from build123d import *

# Parameters (mm, degrees)
BOSS_EXTRUDE1_DEPTH = 76.2
CUT_EXTRUDE1_START  = -3.175
SKETCH2_R           = 3.175
SKETCH2_R_2         = 2.921
CUT_EXTRUDE1_DEPTH  = 0.7874
CUT_EXTRUDE2_START  = -28.321
SKETCH3_R           = 3.175
SKETCH3_R_2         = 2.921
CUT_EXTRUDE2_DEPTH  = 0.7874
CUT_EXTRUDE3_START  = -22.8092
SKETCH3_6_R         = 3.175
SKETCH3_6_R_2       = 2.921
CUT_EXTRUDE3_DEPTH  = 0.7874
CUT_EXTRUDE4_START  = -6.1214
SKETCH3_7_R         = 3.175
SKETCH3_7_R_2       = 2.921
CUT_EXTRUDE4_DEPTH  = 0.7874


with BuildPart() as part:
    # Sketch1 → Boss-Extrude1 (new body)
    with BuildSketch(Plane(origin=(0, 0, 0), x_dir=(1, 0, 0), z_dir=(0, 1, 0))):
        with BuildLine():
            Line((-1, 3.01340754), (-1, 1.81340754))
            Line((-1, 1.81340754), (1, 1.81340754))
            Line((1, 1.81340754), (1, 3.01340754))
            ThreePointArc((1, 3.01340754), (0, -3.175), (-1, 3.01340754))
        make_face()
    extrude(amount=BOSS_EXTRUDE1_DEPTH)

    # Sketch2 → Cut-Extrude1 (cut)
    with BuildSketch(Plane(origin=(0, 76.2, 0), x_dir=(1, 0, 0), z_dir=(0, 1, 0)).offset(CUT_EXTRUDE1_START)):
        Circle(SKETCH2_R)
        Circle(SKETCH2_R_2, mode=Mode.SUBTRACT)
    extrude(amount=CUT_EXTRUDE1_DEPTH, mode=Mode.SUBTRACT)

    # Sketch3 → Cut-Extrude2 (cut)
    with BuildSketch(Plane(origin=(0, 0, 0), x_dir=(0, 0, -1), z_dir=(0, -1, 0)).offset(CUT_EXTRUDE2_START)):
        Circle(SKETCH3_R)
        Circle(SKETCH3_R_2, mode=Mode.SUBTRACT)
    extrude(amount=CUT_EXTRUDE2_DEPTH, mode=Mode.SUBTRACT)

    # Sketch3<6> → Cut-Extrude3 (cut)
    with BuildSketch(Plane(origin=(0, 0, 0), x_dir=(0, 0, -1), z_dir=(0, -1, 0)).offset(CUT_EXTRUDE3_START)):
        Circle(SKETCH3_6_R)
        Circle(SKETCH3_6_R_2, mode=Mode.SUBTRACT)
    extrude(amount=CUT_EXTRUDE3_DEPTH, mode=Mode.SUBTRACT)

    # Sketch3<7> → Cut-Extrude4 (cut)
    with BuildSketch(Plane(origin=(0, 0, 0), x_dir=(0, 0, -1), z_dir=(0, -1, 0)).offset(CUT_EXTRUDE4_START)):
        Circle(SKETCH3_7_R)
        Circle(SKETCH3_7_R_2, mode=Mode.SUBTRACT)
    extrude(amount=CUT_EXTRUDE4_DEPTH, mode=Mode.SUBTRACT)


solid = part.part
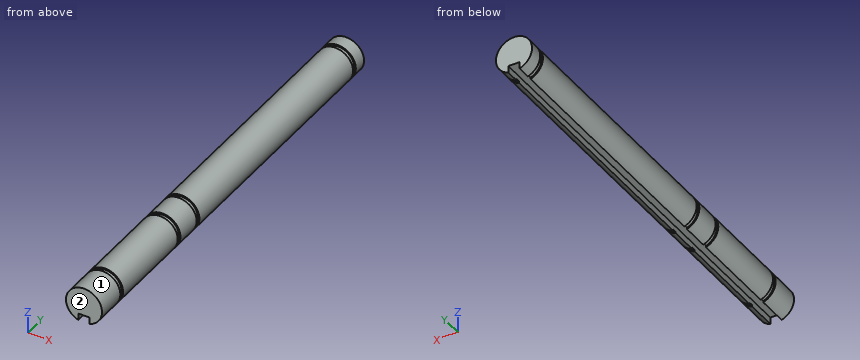
For this review, take the finished solid that the model builds, in its own axes (mm). Face numbers are marked on the shaded views. Coordinates: 2 decimals unless noted, no trailing zeros. Loops run counter-clockwise (first coordinate to the right, second up) from the corner with the lowest first, then second, coordinate; pieces in that order, holes last. Notation, with made-up numbers: (89, 19) - (100, 19) arc R30 ccw to (100, 55) - close; hole circle Ø7 at (31, 87.25). An arc over 180 degrees is marked (long way). Return JSON: item names as keys, results as strings.
Item 1: Insertion check: pin 1 (1.5 mm diameter, centred on x = 2, y = 16.5, fed in from -Z); pin 2 (1.6 mm diameter, centred on x = -0.5, y = 35, fed in from -Z); pin 3 (0.6 mm diameter, centred on y = 45, z = -2.5, fed in from +X). Each pin has a flat end and moves straight along its axis. Give the tip position at first contact, or say it passes through.
Determined:
{"pin 1": "stops at z = -2.92", "pin 2": "stops at z = -3.01", "pin 3": "stops at x = 2.29"}
Item 2: Take a section at A-A (x = 0). Give the boundary of the cut face in (y, z) (3 decimals), then the cut area to 3 significant figures.
Determined:
{"outline": "(0, -1.813) - (76.2, -1.813) - (76.2, 3.175) - (73.812, 3.175) - (73.812, 2.921) - (73.025, 2.921) - (73.025, 3.175) - (28.321, 3.175) - (28.321, 2.921) - (27.534, 2.921) - (27.534, 3.175) - (22.809, 3.175) - (22.809, 2.921) - (22.022, 2.921) - (22.022, 3.175) - (6.121, 3.175) - (6.121, 2.921) - (5.334, 2.921) - (5.334, 3.175) - (0, 3.175) - close", "area": "379 mm2"}
Item 3: Mouldability with a two-part tool opening along X and no side actions: class the marked faces 1 and 2 as pulls with the +X half, pulls with the -X half, needs draft (parallel to the pull), parting line crosses it, or undercut.
Determined:
{"face 1": "parting line crosses it", "face 2": "needs draft"}
Item 4: For line 1 (X direction, y = 31.5, z = -2.25); line 2 (X direction, y = 28, z = 0), list the stretches that pass through material, from the lowest coordinate up.
Determined:
{"line 1": "x = -2.24 to -1, 1 to 2.24", "line 2": "x = -2.92 to 2.92"}
Item 5: Take a section at B-B (y = 13). Give the boundary of the cut face in (x, z) (3 decimals).
Determined:
{"outline": "(-1, -3.013) - (-1, -1.813) - (1, -1.813) - (1, -3.013) arc R3.175 ccw (long way) to start"}
